Check sheet for the drawn part. Datum: minimum x, y, z corner. Units: mm. Coordinates: 2 decimals unless noted, no trailing zeros. Order: outer loops, then holes, each group sorted by start corner. A loop starts at its lowest first (then second) coordinate and runs counter-clockwise, first axis right, second up. Notation, with made-up numbers: (-11, 73) - (39, 73) arc R5 cw to (39, 79) - close; hole circle Ø4 at (13, 56). An arc over 180 degrees is marked (long way). One line per item, written item: value. Start each with the question number.
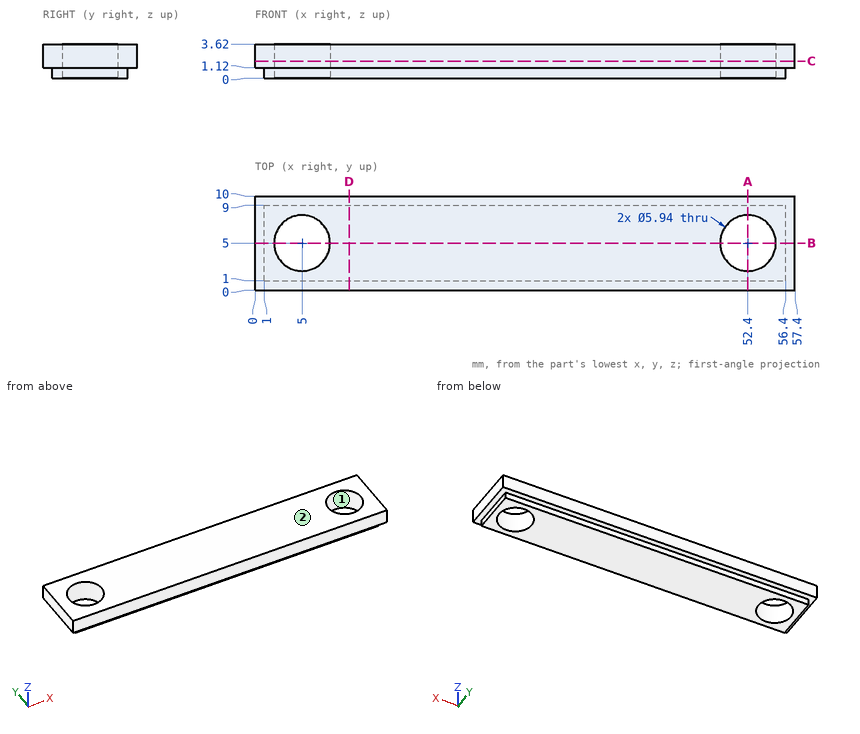
Q1. Release check for a two-part mould opening along X. For the marked faces 1 and 2 record: released by +X, released by -X, zero draft, split by the parting line, or undercut.
Q2. Cross-section at C-C, the plane z = 1.8. Enter the section's corners in (x, y), and give its area (3 significant figures).
Q3. Material ranges on probe 1 along X at (y, z) = (4.75, 0.4); probe 2 along Y at (x, z) = (52.4, 2.1); probe 3 along X at (y, z) = (3, 3.55), recorded low to high.
Q4. Cross-section at B-B, the plane y = 5. Enter the section's corners in (x, z).
Q5. Gauge pin test, flat ends, axial feed: P1, Ø0.9, axis at y = 4.5, z = 1, coming from the +X side; P2, Ø0.6, axis at x = 24.5, z = 0.5, coming from the +Y side; P3, Ø0.6, axis at x = 34, z = 0.5, coming from the -Y side. Record the tip position at first contact, or that the pin passes through.
Q6. Cross-section at A-A, the plane x = 52.4. Enter the section's corners in (y, z), and give its area (3 significant figures).
Q7. Cross-section at D-D, the plane x = 10. Enter the section's corners in (y, z), and give its area (3 significant figures).
Check result:
1. face 1: undercut
1. face 2: zero draft
2. outline: (0, 0) - (57.4, 0) - (57.4, 10) - (0, 10) - close; hole circle Ø5.94 at (5, 5); hole circle Ø5.94 at (52.4, 5)
2. area: 519 mm2
3. probe 1: x = 1 to 2.04, 7.96 to 49.44, 55.36 to 56.4
3. probe 2: y = 0 to 2.03, 7.97 to 10
3. probe 3: x = 0 to 2.8, 7.2 to 50.2, 54.6 to 57.4
4. outline: (0, 1.12) - (1, 1.12) - (1, 0) - (2.03, 0) - (2.03, 3.62) - (0, 3.62) - close; (7.97, 0) - (49.43, 0) - (49.43, 3.62) - (7.97, 3.62) - close; (55.37, 0) - (56.4, 0) - (56.4, 1.12) - (57.4, 1.12) - (57.4, 3.62) - (55.37, 3.62) - close
5. P1: stops at x = 57.4
5. P2: stops at y = 9
5. P3: stops at y = 1
6. outline: (0, 1.12) - (1, 1.12) - (1, 0) - (2.03, 0) - (2.03, 3.62) - (0, 3.62) - close; (7.97, 0) - (9, 0) - (9, 1.12) - (10, 1.12) - (10, 3.62) - (7.97, 3.62) - close
6. area: 12.5 mm2
7. outline: (0, 1.12) - (1, 1.12) - (1, 0) - (9, 0) - (9, 1.12) - (10, 1.12) - (10, 3.62) - (0, 3.62) - close
7. area: 34.0 mm2
